Autodesk Inventor part; units mm, degrees
ref_plane "YZ Plane" through (0, 0, 0) normal (1, 0, 0) x (0, 1, 0)
ref_plane "XZ Plane" through (0, 0, 0) normal (0, 1, 0) x (-1, 0, 0)
ref_plane "XY Plane" through (0, 0, 0) normal (0, 0, 1) x (1, 0, 0)
sketch "Sketch1" plane through (0, 0, 0) normal (0, 1, 0) x (-1, 0, 0)
  line L0 (-50.8, 112.3379) -> (50.8, 112.3379)
  line L1 (50.8, 112.3379) -> (50.8, -112.3378)
  line L2 (50.8, -112.3378) -> (-50.8, -112.3379)
  line L3 (-50.8, -112.3379) -> (-50.8, 112.3379)
  line L4 (-50.8, 112.3379) -> (50.8, -112.3378) construction
  line L5 (50.8, 112.3379) -> (-50.8, -112.3379) construction
  line L6 (-50.8, 92.0813) -> (25.4, 92.0813)
  line L7 (25.4, 92.0813) -> (25.4, -92.0686)
  line L8 (25.4, -92.0686) -> (-50.8, -92.0687)
  line L9 (0, 0) -> (56.1136, 0) construction
  line L10 (76.673, 0) -> (-65.4748, 0)
  line L11 (-31.0246, 99.6379) -> (-31.0246, 0.0063) construction
  line L12 (-31.0246, 0.0063) -> (34.0182, 0.0063) construction
  point P0 (25.4, 0.0063)
  point P1 (-31.0246, -99.6379)
  dimension "d0" = 101.6
  dimension "d56" = 184.15
  dimension "d57" = 76.2
  dimension "d58" = 76.2
  dimension "d60" = 12.7
  dimension "d61" = 12.7
  dimension "d62" = 99.6315
  dimension "d63" = 0
  dimension "d64" = 7.5692
extrude "Extrusion1" add sketch "Sketch1" along normal blind 38.1 contours L0 L1 L10 L7 L6 L3 | L1 L2 L3 L8 L7 L10
fillet "Fillet1" radius 12.7 4 edges at (50.8, 19.05, 112.3379) (-50.8, 19.05, 112.3379) (-50.8, 19.05, -112.3378) (50.8, 19.05, -112.3379)
sketch "Sketch2" plane through (0, 38.1, 0) normal (0, 1, 0) x (1, 0, 0)
  line L0 (-38.1, -112.3379) -> (38.1, -112.3379)
  circle A0 centre (-35.8052, -99.6379) radius 3.3782
  line L1 (-35.8052, -99.6379) -> (-35.8052, 103.5621) construction
  line L2 (-35.8052, -99.6379) -> (40.3948, -99.6379) construction
  line L3 (-35.8052, 103.5621) -> (40.3948, 103.5621) construction
  circle A1 centre (-35.8052, -86.3537) radius 3.3782 construction
  line L4 (-39.1834, -96.2597) -> (-30.0963, -96.2597) construction
  circle A2 centre (-35.8052, -73.0695) radius 3.3782 construction
  circle A3 centre (-35.8052, -59.7853) radius 3.3782 construction
  circle A4 centre (-35.8052, -46.5011) radius 3.3782 construction
  circle A5 centre (-35.8052, -33.2169) radius 3.3782 construction
  circle A6 centre (-35.8052, -19.9327) radius 3.3782 construction
  circle A7 centre (-35.8052, -6.6485) radius 3.3782 construction
  circle A8 centre (-35.8052, 6.6357) radius 3.3782 construction
  circle A9 centre (-35.8052, 19.9199) radius 3.3782 construction
  circle A10 centre (-35.8052, 33.2041) radius 3.3782 construction
  circle A11 centre (-35.8052, 46.4883) radius 3.3782 construction
  circle A12 centre (-35.8052, 59.7725) radius 3.3782 construction
  circle A13 centre (-35.8052, 73.0567) radius 3.3782 construction
  circle A14 centre (-35.8052, 86.3409) radius 3.3782 construction
  circle A15 centre (-35.8052, 99.6251) radius 3.3782 construction
  circle A16 centre (-22.521, -99.6379) radius 3.3782 construction
  circle A17 centre (-9.2368, -99.6379) radius 3.3782 construction
  circle A18 centre (4.0474, -99.6379) radius 3.3782 construction
  circle A19 centre (17.3316, -99.6379) radius 3.3782 construction
  circle A20 centre (30.6158, -99.6379) radius 3.3782 construction
  circle A21 centre (43.9, -99.6379) radius 3.3782 construction
  circle A22 centre (30.6158, 99.6251) radius 3.3782 construction
  circle A23 centre (30.6158, -99.6379) radius 3.3782 construction
  circle A24 centre (-35.8052, 99.6251) radius 3.3782 construction
  circle A25 centre (-35.8052, 33.2041) radius 3.3782 construction
  circle A26 centre (-35.8052, -33.2169) radius 3.3782 construction
  circle A27 centre (-35.8052, -33.2169) radius 3.3782
  circle A28 centre (-35.8052, 33.2041) radius 3.3782
  circle A29 centre (-35.8052, 99.6251) radius 3.3782
  circle A30 centre (30.6158, 99.6251) radius 3.3782
  circle A31 centre (30.6158, -99.6379) radius 3.3782
  point P0 (0, 0)
  point P1 (-35.8052, -23.4379)
  point P2 (-35.8052, 27.3621)
  dimension "d8" = 12.7
  dimension "d9" = 76.2
  dimension "d10" = 127
  dimension "d11" = 203.2
  dimension "d12" = 76.2
  dimension "d13" = 6.7564
  dimension "d22" = 13.2842
  dimension "d25" = 13.2842
  dimension "d30" = 13.2842
  dimension "d33" = 13.2842
  dimension "d38" = 6.7564
  dimension "d39" = 6.7564
  dimension "d40" = 6.7564
  dimension "d41" = 6.7564
  dimension "d42" = 6.7564
  dimension "d43" = 6.7564
  dimension "d44" = 6.7564
  dimension "d45" = 6.7564
  dimension "d46" = 6.7564
extrude "Extrusion4" cut sketch "Sketch2" against normal through all
equation "\"d25\" = d22"
equation "\"d30\" = d22"
equation "\"d33\" = d22"
properties part number "FBH!"
Input: part model. Units: mm. Frame: model coordinates. A direction names the side the tool comes from. Give positions to 0.01 mm unless a question says otherwise; leave off trailing zeros. Order: outer loops, then holes, each group sorted by start corner. A loop starts at its lowest first (then second) coordinate and runs counter-clockwise, first axis right, second up. Notation, with made-up numbers: (36.5, 78) - (73.5, 78) arc R9 ccw to (73.5, 95) - close; hole circle Ø3 at (-38, -8). An arc over 180 degrees is marked (long way). Write each question's results on one line, items separated by ' | '.
Item 1: Draft query along X for faces 1 (the cylindrical face through (29.88, 19.32, -96.33)), 2 (the flat face through (50.8, 19, 96)), 3 (the flat face through (1, 19, 112.338)). Return one class per face: released by +X, released by -X, zero draft, split by the parting line, or undercut.
A:
face 1: undercut | face 2: released by +X | face 3: zero draft
Item 2: Material intervals for line 1 along Z through (x, y) = (31, 9); line 2 along Z through (x, y) = (-4.5, 11.5); line 3 along X through (y, z) = (21, -97), sorted ascending.
A:
line 1: z = -112.34 to -102.98, -96.27 to -92.07, 92.08 to 96.28, 102.99 to 112.34 | line 2: z = -112.34 to -92.07, 92.08 to 112.34 | line 3: x = -50.8 to -37.93, -33.68 to 28.49, 32.74 to 50.8
Item 3: Section A-A (x = 17). Return loops of the section in (y, z), and give its area (3 significant figures).
A:
outline: (0, -112.34) - (38.1, -112.34) - (38.1, -92.07) - (0, -92.07) - close; (0, 92.08) - (38.1, 92.08) - (38.1, 112.34) - (0, 112.34) - close | area: 1,540 mm^2
Item 4: Access query for faces 4 (the cylindrical face through (47, 19.3, 108.7)), 5 (the flat face through (-25.4, 19, 1)). Directions: +Z, -Z, +X, -X, +Y, -Y. A direction counts if a zero-diameter tool reaches every point of the face in a straight line with its end or side. Return the directions, or none.
A:
face 4: +Z, +X, +Y, -Y | face 5: +X, +Y, -Y
Item 5: Contact query for a flat-ended pin moving along its axis: pin 1 Ø11.5 at (y, z) = (13, -19) entering from +X. Output: stop coordinate, or through.
A:
pin 1: stops at x = -25.4
Item 6: Section C-C (z = 49.5). Return loops of the section in (x, y), and give its area (3 significant figures).
A:
outline: (-50.8, 0) - (-25.4, 0) - (-25.4, 38.1) - (-50.8, 38.1) - close | area: 968 mm^2
Item 7: Section B-B (y = 10). Return loops of the section in (x, z).
A:
outline: (-50.8, -99.64) arc R12.7 ccw to (-38.1, -112.34) - (38.1, -112.34) arc R12.7 ccw to (50.8, -99.64) - (50.8, -92.07) - (-25.4, -92.07) - (-25.4, 92.08) - (50.8, 92.08) - (50.8, 99.64) arc R12.7 ccw to (38.1, 112.34) - (-38.1, 112.34) arc R12.7 ccw to (-50.8, 99.64) - close; hole circle Ø6.76 at (-35.81, -99.63); hole circle Ø6.76 at (-35.81, -33.2); hole circle Ø6.76 at (-35.81, 33.22); hole circle Ø6.76 at (-35.81, 99.64); hole circle Ø6.76 at (30.62, -99.63); hole circle Ø6.76 at (30.62, 99.64)
